Design review of the part shown in the three views and the two pictorial views. Dimensions are in mm from the part's minimum x, y and z. A direction names the side the tool comes from. Give positions to 0.01 mm unless a question says otherwise; leave off trailing zeros. Loops run counter-clockwise (first coordinate to the right, second up) from the corner with the lowest first, then second, coordinate; pieces in that order, holes last. Notation, with made-up numbers: (12, 38) - (19, 38) arc R24 ccw to (19, 74) - close; hole circle Ø6 at (79.25, 87). An arc over 180 degrees is marked (long way). Return JSON: item names as keys, results as strings. Group by question number.
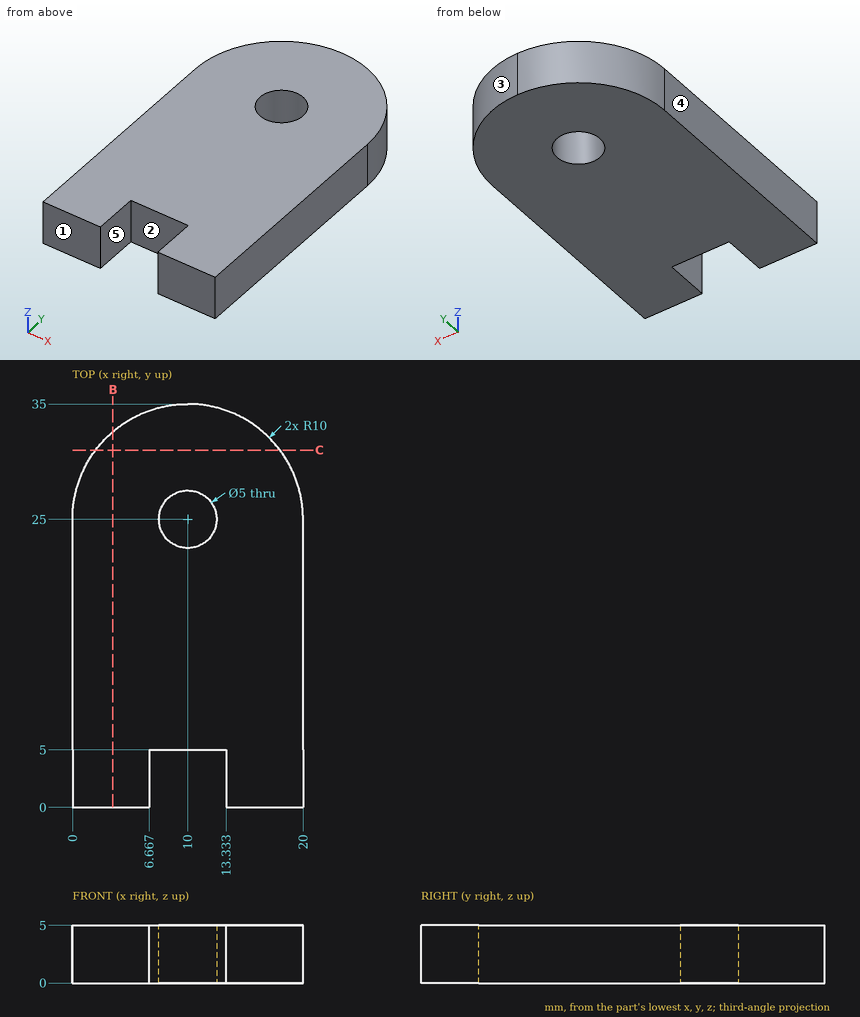
Item 1: For P1, Ø4.5, axis at x = 10, y = 25, coming from the +Z side; P2, Ø4, axis at x = 17, y = 29.5, coming from the -Z side; P3, Ø1, axis at y = 29.5, z = 3.5, coming from the +X side (1 decimal); P4, Ø1.5, axis at x = 6.5, z = 3, coming from the +Y side (1 decimal), all flat-tipped, find the tip position at first contact; note any pin that passes through.
Item 2: For L1, parallel to Y at x = 10, z = 1.6; L2, parallel to Y at x = 11.5, z = 1.3; L3, parallel to X at y = 24, z = 3.9, list the stretches that pass through material, from the lowest coordinate up. Write a range as from..to.
Item 3: Mouldability with a two-part tool opening along X and no side actions: class the marked faces 3, 4 and 5 as +X half, -X half, draft (parallel to the pull), parting line (faces both ways), or undercut.
Item 4: Tool access review of the marked faces 1 and 2: name each direction out of +Z, -Z, +X, -X, +Y, -Y from which nothing blocks a thin tool from reaching the whole face with its end or side.
Item 5: Take a section at B-B (x = 3.5). State the section outline as (y, z) points.
Item 6: Take a section at C-C (y = 31). State the section outline as (x, z) points, then the cut area to 3 significant figures.
Check sheet entries:
{
 "1": {"P1": "passes through", "P2": "stops at z = 0", "P3": "stops at x = 19.2", "P4": "stops at y = 34.6"},
 "2": {"L1": "y = 5..22.5, 27.5..35", "L2": "y = 5..23, 27..34.89", "L3": "x = 0..7.71, 12.29..20"},
 "3": {"face 3": "+X half", "face 4": "-X half", "face 5": "undercut"},
 "4": {"face 1": "+Z, -Z, +X, -X, -Y", "face 2": "+Z, -Z, -Y"},
 "5": {"outline": "(0, 0) - (32.6, 0) - (32.6, 5) - (0, 5) - close"},
 "6": {"outline": "(2, 0) - (18, 0) - (18, 5) - (2, 5) - close", "area": "80.0 mm^2"}
}
